```python
from build123d import *

# Parameters (mm, degrees)
F1_DEPTH = 25.4
F2_DEPTH = 12.7
F3_R     = 6.35
F4_DEPTH = 38.1


with BuildPart() as f1:
    # F0 (on Front) → F1 (new body)
    with BuildSketch(Plane.XZ):
        with BuildLine():
            ThreePointArc((44.45, 55.88), (42.218154, 61.268154), (36.83, 63.5))
            Line((36.83, 63.5), (-36.83, 63.5))
            ThreePointArc((-36.83, 63.5), (-42.218154, 61.268154), (-44.45, 55.88))
            Line((-44.45, 55.88), (-44.45, -55.88))
            ThreePointArc((-44.45, -55.88), (-42.218154, -61.268154), (-36.83, -63.5))
            Line((-36.83, -63.5), (36.83, -63.5))
            ThreePointArc((36.83, -63.5), (42.218154, -61.268154), (44.45, -55.88))
            Line((44.45, -55.88), (44.45, 55.88))
        make_face()
        with BuildLine():
            Line((-31.75, 57.15), (31.75, 57.15))
            ThreePointArc((31.75, 57.15), (36.240128, 55.290128), (38.1, 50.8))
            Line((38.1, 50.8), (38.1, -50.8))
            ThreePointArc((38.1, -50.8), (36.240128, -55.290128), (31.75, -57.15))
            Line((31.75, -57.15), (-31.75, -57.15))
            ThreePointArc((-31.75, -57.15), (-36.240128, -55.290128), (-38.1, -50.8))
            Line((-38.1, -50.8), (-38.1, 50.8))
            ThreePointArc((-38.1, 50.8), (-36.240128, 55.290128), (-31.75, 57.15))
        make_face(mode=Mode.SUBTRACT)
        with BuildLine():
            ThreePointArc((38.1, 50.8), (36.240128, 55.290128), (31.75, 57.15))
            Line((31.75, 57.15), (-31.75, 57.15))
            ThreePointArc((-31.75, 57.15), (-36.240128, 55.290128), (-38.1, 50.8))
            Line((-38.1, 50.8), (-38.1, -50.8))
            ThreePointArc((-38.1, -50.8), (-36.240128, -55.290128), (-31.75, -57.15))
            Line((-31.75, -57.15), (31.75, -57.15))
            ThreePointArc((31.75, -57.15), (36.240128, -55.290128), (38.1, -50.8))
            Line((38.1, -50.8), (38.1, 50.8))
        make_face()
    extrude(amount=F1_DEPTH)

    # F0 (on Front) → F2 (cut)
    with BuildSketch(Plane.XZ):
        with BuildLine():
            ThreePointArc((38.1, 50.8), (36.240128, 55.290128), (31.75, 57.15))
            Line((31.75, 57.15), (-31.75, 57.15))
            ThreePointArc((-31.75, 57.15), (-36.240128, 55.290128), (-38.1, 50.8))
            Line((-38.1, 50.8), (-38.1, -50.8))
            ThreePointArc((-38.1, -50.8), (-36.240128, -55.290128), (-31.75, -57.15))
            Line((-31.75, -57.15), (31.75, -57.15))
            ThreePointArc((31.75, -57.15), (36.240128, -55.290128), (38.1, -50.8))
            Line((38.1, -50.8), (38.1, 50.8))
        make_face()
    extrude(amount=F2_DEPTH, mode=Mode.SUBTRACT)

    # F3 (on face) → F4 (join)
    with BuildSketch(Plane.XZ.offset(25.4)):
        with Locations((-36.83, 55.88)):
            Circle(F3_R)
        with Locations((36.83, 55.88)):
            Circle(F3_R)
        with Locations((-36.83, -55.88)):
            Circle(F3_R)
        with Locations((36.83, -55.88)):
            Circle(F3_R)
    extrude(amount=F4_DEPTH)


solid = f1.part
```
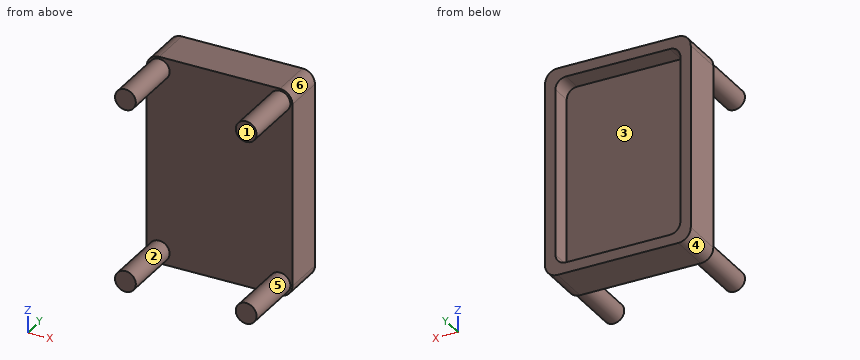
Input: part model. Units: mm. Frame: model coordinates. Face numbers are marked on the shaded views. A direction names the side the tool comes from. Give positions to 0.01 mm unless a question says otherwise; leave off trailing zeros. Write each loop counter-clockwise with the first axis right and the second up, starting at its lowest first coordinate (ties: lowest second). Pieces come first, ordered by that corner, then holes. Notation, with made-up numbers: (-33, 60) - (-8, 60) arc R27 cw to (-8, 98) - close; hole circle Ø11 at (-35, 70.25). An arc over 180 degrees is marked (long way). Write item = value, one per line. Start each with the question number.
1. Section query A-A, the plane z = -35. Output: boundary loops of the cut face in (x, y), then the cut area to 3 significant figures.
2. Access query for the marked faces 1, 2 and 3. Directions: +Z, -Z, +X, -X, +Y, -Y. A direction counts if a zero-diameter tool reaches every point of the face in a straight line with its end or side. Return the directions, or none.
3. Mould query, pull axis X, two halves, no side actions, for the marked faces 4, 5 and 6. Classes: released by +X, released by -X, zero draft, split by the parting line, or undercut.
4. Section query B-B, the plane x = -20.5. Output: boundary loops of the cut face in (y, z).
5. Ray query, L1, parallel to Z at x = -18, y = -11.5; L2, parallel to Y at x = -4, z = 26. Return the intervals inside material, ascending.
6. Section query C-C, the plane y = -34. Output: boundary loops of the cut face in (x, z).
7. First-contact query: pin 1 Ø5 at (x, z) = (-28.5, -29.5) entering from -Y; pin 2 Ø8 at (x, z) = (-3, -14) entering from +Y. Flat tips, straight axial feed; report the tip coordinate or a pass-through.
Check sheet entries:
q1.outline = (-44.45, -25.4) - (44.45, -25.4) - (44.45, 0) - (38.1, 0) - (38.1, -12.7) - (-38.1, -12.7) - (-38.1, 0) - (-44.45, 0) - close
q1.area = 1,290 mm2
q2.face_1 = +Z, -Z, +X, -X, -Y
q2.face_2 = -Y
q2.face_3 = +Y
q3.face_4 = released by -X
q3.face_5 = undercut
q3.face_6 = released by +X
q4.outline = (-25.4, -63.5) - (0, -63.5) - (0, -57.15) - (-12.7, -57.15) - (-12.7, 57.15) - (0, 57.15) - (0, 63.5) - (-25.4, 63.5) - close
q5.L1 = -63.5 to -57.15, 57.15 to 63.5
q5.L2 = -25.4 to -12.7
q6.outline = circle Ø12.7 at (-36.83, -55.88); circle Ø12.7 at (-36.83, 55.88); circle Ø12.7 at (36.83, -55.88); circle Ø12.7 at (36.83, 55.88)
q7.pin_1 = -25.4
q7.pin_2 = -12.7
